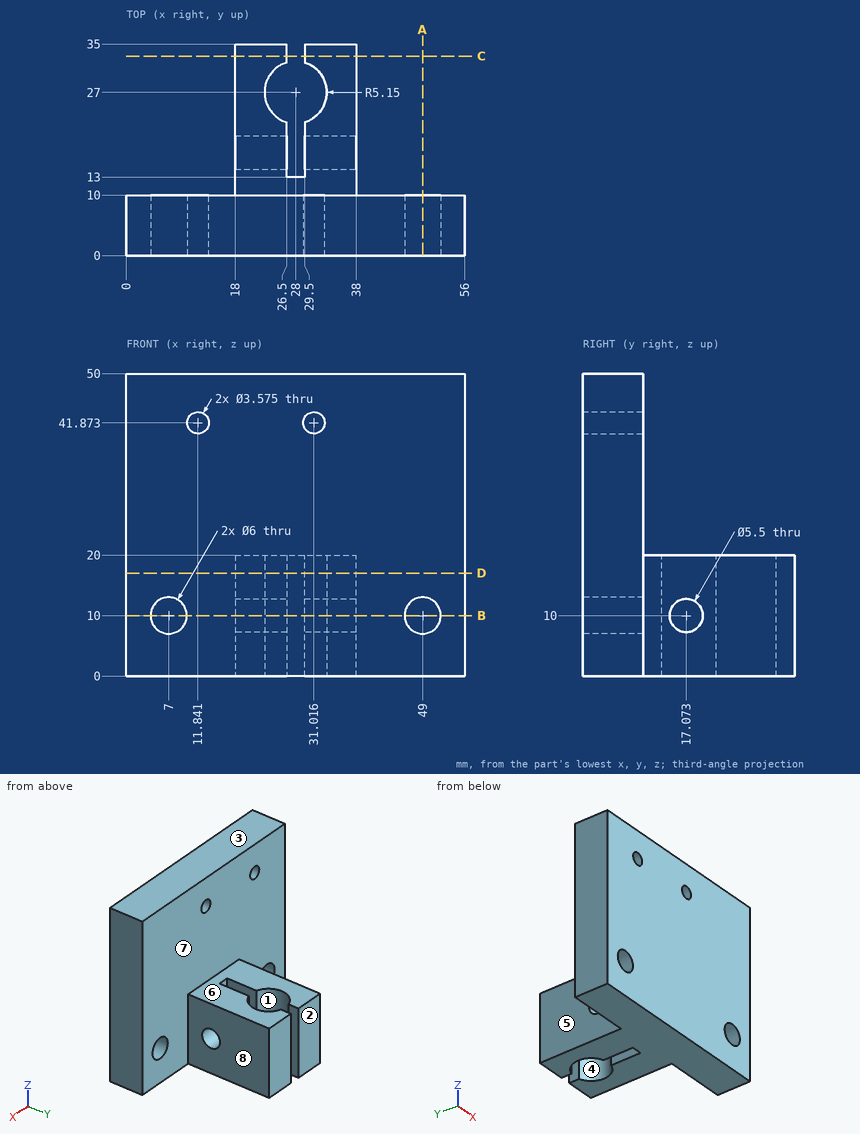
Geometry check sheet. Reference: drawing and pictorial views, mm from the part's lowest x, y, z. A direction names the side the tool comes from. Give positions to 0.01 mm unless a question says otherwise; leave off trailing zeros. Order: outer loops, then holes, each group sorted by start corner. A loop starts at its lowest first (then second) coordinate and runs counter-clockwise, first axis right, second up. Notation, with made-up numbers: (-27, 10.5) -> (7, 10.5) arc R25 ccw to (7, 29.5) -> close; hole circle Ø2 at (-32.5, 85). An arc over 180 degrees is marked (long way). Write each question's results on one line, items separated by ' | '. Start each with the question number.
(1) Mould release check, pull along Y, two halves, no side actions. Record for the marked faces 1, 2 and 3: pulls with the +Y half, pulls with the -Y half, needs draft (parallel to the pull), parting line crosses it, or undercut.
(2) Sectioned sample at B-B (z = 10). Give the number of separate pieces and of enclosed holes in the cut face.
(3) Sectioned sample at A-A (x = 49). Enter the section's corners in (y, z), plus the area to 3 significant figures.
(4) Scan lines: line 1 (X direction, y = 14, z = 15.5); line 2 (X direction, y = 7.5, z = 7.5) (1 decimal); line 3 (Y direction, x = 9, z = 25). Record each from-to range of solid material in increasing order.
(5) Access from +Z, -Z, +X, -X, +Y, -Y to the whole of each face (thin tool, end or side, straight path). Record for the marked faces 4, 5, 6, 7 and 8.
(6) Gauge pin test, flat ends, axial feed: P1, Ø10, axis at x = 49, z = 29.5, coming from the +Y side; P2, Ø10, axis at y = 17, z = 14.5, coming from the +X side; P3, Ø0.9, axis at y = 34, z = 6.5, coming from the -X side. Record the tip position at first contact, or that the pin passes through.
(7) Sectioned sample at C-C (y = 33). Enter the section's corners in (x, z).
(8) Sectioned sample at D-D (z = 17). Enter the section's corners in (x, y).
Answer below:
1) face 1: undercut | face 2: pulls with the +Y half | face 3: needs draft
2) separate pieces: 5 | enclosed holes: 0
3) outline: (0, 0) -> (10, 0) -> (10, 7) -> (0, 7) -> close; (0, 13) -> (10, 13) -> (10, 50) -> (0, 50) -> close | area: 440 mm2
4) line 1: 18 to 26.5, 29.5 to 38 | line 2: 0 to 5.3, 8.7 to 47.3, 50.7 to 56 | line 3: 0 to 10
5) face 4: +Z, -Z | face 5: +Z, -Z, -X, +Y | face 6: +Z, +X, -X, +Y | face 7: +Z, +Y | face 8: +Z, -Z, +X, +Y
6) P1: y = 10 | P2: x = 38 | P3: x = 18
7) outline: (18, 0) -> (26.5, 0) -> (26.5, 20) -> (18, 20) -> close; (29.5, 0) -> (38, 0) -> (38, 20) -> (29.5, 20) -> close
8) outline: (0, 0) -> (56, 0) -> (56, 10) -> (38, 10) -> (38, 35) -> (29.5, 35) -> (29.5, 31.93) arc R5.15 cw to (29.5, 22.07) -> (29.5, 13) -> (26.5, 13) -> (26.5, 22.07) arc R5.15 cw to (26.5, 31.93) -> (26.5, 35) -> (18, 35) -> (18, 10) -> (0, 10) -> close
